Here's how the part is built. I have some questions about the finished solid (model axes, mm). A direction names the side the tool comes from. Give positions to 0.01 mm unless a question says otherwise; leave off trailing zeros. Loops run counter-clockwise (first coordinate to the right, second up) from the corner with the lowest first, then second, coordinate; pieces in that order, holes last. Notation, with made-up numbers: (21, 34.5) -> (79, 34.5) arc R19 ccw to (79, 56.5) -> close; hole circle Ø9 at (58, 67). An arc over 180 degrees is marked (long way). Answer in a Markdown table with one row per item. Add a question column.
Item 1: If we section it at C-C (x = 1.5): Write out the boundary of the cut face in (y, z), then the cut area to 3 significant figures.
Item 2: If I drill on line 1 (X direction, y = -69, z = 4); line 2 (Z direction, x = -37, y = -54.5); line 3 (X direction, y = -33, z = 21), over which ranges is the centre line in solid material (lowest first)?
Item 3: Which directions (+Z, -Z, +X, -X, +Y, -Y) give clear straight access to the entire face, cutting with the end or side of a thin tool? Please do faces 1 (the face through (-19, -25.4, -32)), 2 (the face through (-53.38, -38, 13)), 3 (the face through (-36.06, -62, 13)), 4 (the face through (4, -34.498, 13)), 5 (the face through (0, -17, 8)).
Item 4: If we section it at A-A (y = -62): Write out the boundary of the cut face in (x, z), then the cut area to 3 significant figures.
Item 5: If we section it at D-D (y = -22.5): Write out the boundary of the cut face in (x, z), then the cut area to 3 significant figures.
Item 6: For P1, Ø6.5, axis at x = 5, z = 7, coming from the +Y side; P2, Ø10, axis at y = -9.5, z = 1.5, coming from the +X side; P3, Ø1.5, axis at y = -59.5, z = 12, coming from the +X side, each with a flat end and sliding along its axis, tell me the tip position at first contact or that it passes through.
Item 7: If we section it at B-B (z = 18.5): Write out the boundary of the cut face in (x, y).
Item 8: We'd pull the mould along X, two halves only. Please class faces 6 (the face through (-23.703, -35.495, 12.522)), 7 (the face through (9, -13, -8.092)), 8 (the face through (7.95, -56, 13)), 9 (the face through (-18.67, -12.52, -64.62)): released by +X, released by -X, zero draft, split by the parting line, or undercut.
```python
from build123d import *

# Parameters (mm, degrees)
F1_DEPTH = 25.4
F3_DEPTH = 25.4


# Not quite as in the source:
# - ends of sketch curves that miss each other by under 0.0002 mm in the source are joined


with BuildPart() as f1:
    # F0 (on Front) → F1 (new body)
    with BuildSketch(Plane.XZ):
        with BuildLine():
            Line((0, 0), (-53.9480485022, 0))
            Line((-53.9480485022, 0), (-53.9480485022, -41.0289131105))
            ThreePointArc((-53.9480485022, -41.0289131105), (-18.0300064385, -64.6250791293), (17.8880356252, -41.0289131105))
            Line((17.8880356252, -41.0289131105), (17.8880356252, -8.0922106281))
            Line((17.8880356252, -8.0922106281), (0, -8.0922106281))
            Line((0, -8.0922106281), (0, 0))
        make_face()
    extrude(amount=F1_DEPTH)

    # F2 (on Top) → F3 (join)
    with BuildSketch(Plane.XY):
        with BuildLine():
            Line((0, -34.4983525574), (0, -25.6963036954))
            Line((0, -25.6963036954), (0, 0))
            Line((0, 0), (-53.380176425, 0))
            Line((-53.380176425, 0), (-53.380176425, -25.9802397341))
            Line((-53.380176425, -25.9802397341), (-53.380176425, -76.2371048331))
            Line((-53.380176425, -76.2371048331), (-36.0600091517, -76.2371048331))
            Line((-36.0600091517, -76.2371048331), (-36.0600091517, -48.1273345649))
            ThreePointArc((-36.0600091517, -48.1273345649), (-23.424807936, -35.4921333492), (-10.7896067202, -48.1273345649))
            Line((-10.7896067202, -48.1273345649), (-10.7896067202, -76.2371048331))
            Line((-10.7896067202, -76.2371048331), (7.9502388835, -76.2371048331))
            Line((7.9502388835, -76.2371048331), (7.9502388835, -34.4983525574))
            Line((7.9502388835, -34.4983525574), (0, -34.4983525574))
        make_face()
    extrude(amount=F3_DEPTH)


solid = f1.part
```
Recorded:
| question | item | result |
|---|---|---|
| 1 | outline | (-76.24, 0) -> (-34.5, 0) -> (-34.5, 25.4) -> (-76.24, 25.4) -> close; (-25.4, -59.4) -> (0, -59.4) -> (0, -8.09) -> (-25.4, -8.09) -> close |
| 1 | area | 2,360 mm^2 |
| 2 | line 1 | x = -53.38 to -36.06, -10.79 to 7.95 |
| 2 | line 2 | z = 0 to 25.4 |
| 2 | line 3 | x = -53.38 to 0 |
| 3 | face 1 | -Z, +X, -X, -Y |
| 3 | face 2 | +Z, -X, +Y, -Y |
| 3 | face 3 | +Z, -Z, -Y |
| 3 | face 4 | +Z, -Z, +X, +Y |
| 3 | face 5 | +Z, +X, +Y |
| 4 | outline | (-53.38, 0) -> (-36.06, 0) -> (-36.06, 25.4) -> (-53.38, 25.4) -> close; (-10.79, 0) -> (7.95, 0) -> (7.95, 25.4) -> (-10.79, 25.4) -> close |
| 4 | area | 916 mm^2 |
| 5 | outline | (-53.95, -41.03) arc R39.14 ccw to (17.89, -41.03) -> (17.89, -8.09) -> (0, -8.09) -> (0, 25.4) -> (-53.38, 25.4) -> (-53.38, 0) -> (-53.95, 0) -> close |
| 5 | area | 5,380 mm^2 |
| 6 | P1 | stops at y = -34.5 |
| 6 | P2 | stops at x = 0 |
| 6 | P3 | stops at x = 7.95 |
| 7 | outline | (-53.38, -76.24) -> (-36.06, -76.24) -> (-36.06, -48.13) arc R12.64 cw to (-10.79, -48.13) -> (-10.79, -76.24) -> (7.95, -76.24) -> (7.95, -34.5) -> (0, -34.5) -> (0, 0) -> (-53.38, 0) -> close |
| 8 | face 6 | undercut |
| 8 | face 7 | zero draft |
| 8 | face 8 | released by +X |
| 8 | face 9 | split by the parting line |
